Can you work these out from the model? Positions are in its coordinate system, mm. Face numbers are marked on the shaded views. Give positions to 0.01 mm unless a question says otherwise; leave off trailing zeros. Loops run counter-clockwise (first coordinate to the right, second up) from the corner with the lowest first, then second, coordinate; pieces in that order, holes last. Notation, with made-up numbers: M 88,-19.75 L 118,-19.75 A10 cw 118,-14.75 Z; hole C 63.25,31.25 d1. An arc over 180 degrees is marked long. Put each result on its own line as item: value. Start each with the question number.
1) Imagine slicing it at B-B (z = 14.75). Write out the boundary of the cut face in (x, y), then the cut area to 3 significant figures.
2) Imagine slicing it at C-C (x = 507.5). Write out the boundary of the cut face in (y, z), then the cut area to 3 significant figures.
3) Please list where these lines run through material, in increasing order: line 1 along X through (y, z) = (458, 22); line 2 along Z through (x, y) = (553.5, 337.5); line 3 along Y through (x, z) = (211, 23.25). Write a range as from..to.
4) Imagine slicing it at A-A (y = 211). Write out the boundary of the cut face in (x, z).
5) For P1, Ø7, axis at x = 1485, z = 23.5, coming from the +Y side; P2, Ø3, axis at x = 391, y = 484, coming from the +Z side; P3, Ø1, axis at x = 1468.5, y = 458, coming from the -Z side; P4, Ø7, axis at x = 226, z = 22, coming from the +Y side, each with a flat end and sliding along its axis, tell me the tip position at first contact or that it passes through.
6) Imagine slicing it at D-D (x = 722). Write out the boundary of the cut face in (y, z), then the cut area to 3 significant figures.
7) If we mould it in two halves opening along Y, with no side actions, what happens to the marked faces 1, 2 and 3? For each: +Y half, -Y half, draft (parallel to the pull), parting line (faces both ways), or undercut.
from build123d import *

# Parameters (mm, degrees)
F1_DEPTH = 25.4
F3_DEPTH = 6.35


with BuildPart() as f1:
    # F0 (on Top) → F1 (new body)
    with BuildSketch(Plane.XY):
        with BuildLine():
            Line((0, 762), (0, 0))
            Line((0, 0), (304.8, 0))
            ThreePointArc((304.8, 0), (838.2, 96.393458), (1371.6, 0))
            Line((1371.6, 0), (1676.4, 0))
            Line((1676.4, 0), (1676.4, 762))
            ThreePointArc((1676.4, 762), (838.2, 921.214454), (0, 762))
        make_face()
    extrude(amount=F1_DEPTH)

    # F2 (on face) → F3 (cut)
    with BuildSketch(Plane.XY.offset(25.4)):
        with BuildLine():
            Line((1385.197187, 76.200001), (1600.199999, 76.200001))
            Line((1600.199999, 76.200001), (1600.199999, 709.47867))
            ThreePointArc((1600.199999, 709.47867), (1243.921895, 807.449657), (876.299999, 844.68598))
            Line((876.299999, 844.68598), (876.299999, 172.139823))
            ThreePointArc((876.299999, 172.139823), (1134.655379, 144.892822), (1385.197187, 76.200001))
        make_face()
        with BuildLine():
            Line((76.200001, 709.47867), (76.200001, 76.200001))
            Line((76.200001, 76.200001), (291.202813, 76.200001))
            ThreePointArc((291.202813, 76.200001), (541.744621, 144.892822), (800.100001, 172.139823))
            Line((800.100001, 172.139823), (800.100001, 844.68598))
            ThreePointArc((800.100001, 844.68598), (432.478105, 807.449657), (76.200001, 709.47867))
        make_face()
    extrude(amount=-F3_DEPTH, mode=Mode.SUBTRACT)


solid = f1.part
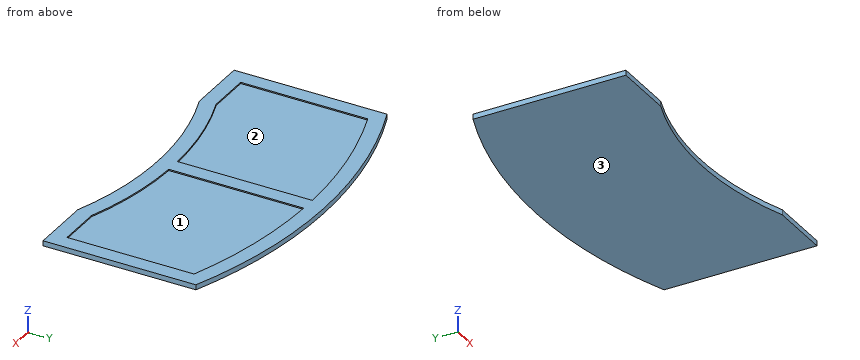
Recorded:
1. outline: M 0,0 L 304.8,0 A1524 cw 1371.6,0 L 1676.4,0 L 1676.4,762 A2286 ccw 0,762 Z
1. area: 1,390,000 mm²
2. outline: M 60.08,0 L 897.17,0 L 897.17,25.4 L 820.13,25.4 L 820.13,19.05 L 138.05,19.05 L 138.05,25.4 L 60.08,25.4 Z
2. area: 16,900 mm²
3. line 1: 0..76.2, 800.1..876.3, 1600.2..1676.4
3. line 2: 0..19.05
3. line 3: 0..76.2, 754.14..833.49
4. outline: M 0,0 L 1676.4,0 L 1676.4,25.4 L 1600.2,25.4 L 1600.2,19.05 L 876.3,19.05 L 876.3,25.4 L 800.1,25.4 L 800.1,19.05 L 76.2,19.05 L 76.2,25.4 L 0,25.4 Z
5. P1: y = 828.83
5. P2: z = 19.05
5. P3: z = 0
5. P4: y = 838.68
6. outline: M 91.96,0 L 918.26,0 L 918.26,25.4 L 841.96,25.4 L 841.96,19.05 L 168.37,19.05 L 168.37,25.4 L 91.96,25.4 Z
6. area: 16,700 mm²
7. face 1: undercut
7. face 2: undercut
7. face 3: draft
